from build123d import *

# Parameters (mm, degrees)
F0_W      = 189.7254064679
F0_H      = 125.3468897194
F1_DEPTH  = 3.81
F2_W      = 6.9400146604
F2_H      = 125.3468897194
F3_DEPTH  = 50.8
F4_W      = 7.941737771
F4_H      = 125.3468897194
F5_DEPTH  = 50.8
F6_W      = 181.0236349702
F6_H      = 7.8539922833
F7_DEPTH  = 177.8
F8_W      = 6.9400146604
F8_H      = 66.6004410014
F9_DEPTH  = 50.8
F10_W     = 6.9400146604
F10_H     = 25.5400016904
F11_DEPTH = 76.2
F12_W     = 7.941737771
F12_H     = 58.746448718
F13_DEPTH = 50.8
F14_W     = 6.1799809337
F14_H     = 15.7597959042
F15_DEPTH = 76.2
F16_W     = 189.6112561226
F16_H     = 127.5956835598
F17_DEPTH = 3.302
F18_W     = 1.9466541708
F18_H     = 54.61
F19_DEPTH = 117.602
F20_W     = 11.5141570568
F20_H     = 125.3468897194
F21_DEPTH = 127
F22_W     = 10.0032910705
F22_H     = 125.3468897194
F23_DEPTH = 127
F24_W     = 178.803190589
F24_H     = 6.9889426231
F25_DEPTH = 127


with BuildPart() as f1:
    # F0 (on Top) → F1 (new body)
    with BuildSketch(Plane.XY):
        with Locations((-30.9122316539, 52.4606974795)):
            Rectangle(F0_W, F0_H)
    extrude(amount=F1_DEPTH)

    # F2 (on face) → F3 (join)
    with BuildSketch(Plane.XY.offset(3.81)):
        with Locations((-122.3049275577, 52.4606974795)):
            Rectangle(F2_W, F2_H)
    extrude(amount=F3_DEPTH)

    # F4 (on face) → F5 (join)
    with BuildSketch(Plane.XY.offset(3.81)):
        with Locations((59.9796026945, 52.4606974795)):
            Rectangle(F4_W, F4_H)
    extrude(amount=F5_DEPTH)

    # F6 (on face) → F7 (join)
    with BuildSketch(Plane.XY.offset(3.81)):
        with Locations((-28.3231027424, 111.2071461976)):
            Rectangle(F6_W, F6_H)
    extrude(amount=F7_DEPTH)

    # F8 (on face) → F9 (join)
    with BuildSketch(Plane.XY.offset(54.61)):
        with Locations((-122.3049275577, 81.8339218386)):
            Rectangle(F8_W, F8_H)
    extrude(amount=F9_DEPTH)

    # F10 (on face) → F11 (join)
    with BuildSketch(Plane.XY.offset(105.41)):
        with Locations((-122.3049275577, 102.364141494)):
            Rectangle(F10_W, F10_H)
    extrude(amount=F11_DEPTH)

    # F12 (on face) → F13 (join)
    with BuildSketch(Plane.XY.offset(54.61)):
        with Locations((59.9796026945, 77.9069256969)):
            Rectangle(F12_W, F12_H)
    extrude(amount=F13_DEPTH)

    # F14 (on face) → F15 (join)
    with BuildSketch(Plane.XY.offset(105.41)):
        with Locations((59.0987242758, 99.4002521038)):
            Rectangle(F14_W, F14_H)
    extrude(amount=F15_DEPTH)

    # F16 (on face) → F17 (join)
    with BuildSketch(Plane.XY.offset(54.61)):
        with Locations((-30.9693068266, 53.5850943998)):
            Rectangle(F16_W, F16_H)
    extrude(amount=F17_DEPTH)

    # F18 (on face) → F19 (join)
    with BuildSketch(Plane.XZ.offset(-107.2801500559)):
        with Locations((-30.4397661239, 27.305)):
            Rectangle(F18_W, F18_H)
    extrude(amount=F19_DEPTH)

    # F20 (on face) → F21 (join)
    with BuildSketch(Plane(origin=(0, 0, 0), x_dir=(1, 0, 0), z_dir=(0, 0, -1))):
        with Locations((-120.0178563595, -52.4606974795)):
            Rectangle(F20_W, F20_H)
    extrude(amount=F21_DEPTH)

    # F22 (on face) → F23 (join)
    with BuildSketch(Plane(origin=(0, 0, 0), x_dir=(1, 0, 0), z_dir=(0, 0, -1))):
        with Locations((58.9488260448, -52.4606974795)):
            Rectangle(F22_W, F22_H)
    extrude(amount=F23_DEPTH)

    # F24 (on face) → F25 (join)
    with BuildSketch(Plane(origin=(0, 0, 0), x_dir=(1, 0, 0), z_dir=(0, 0, -1))):
        with Locations((-35.4544147849, -111.6396710277)):
            Rectangle(F24_W, F24_H)
    extrude(amount=F25_DEPTH)


solid = f1.part
Could you check a few things on this model? Use its own coordinates, in mm. A direction names the side the tool comes from. Give positions to 0.01 mm unless a question says otherwise; leave off trailing zeros. Order: outer loops, then holes, each group sorted by start corner. A loop starts at its lowest first (then second) coordinate and runs counter-clockwise, first axis right, second up.
Item 1: I need wall thicknesses on line 1 (X direction, y = 107, z = 20); line 2 (Z direction, x = 24, y = 67); line 3 (X direction, y = 39.5, z = -38.5). Which ranges of each line are inside material? Lowest first, please.
Item 2: If we mould it in two halves opening along Z, with no side actions, what happens to faces 6 (the face through (-31.413, 49, 33)), 7 (the face through (-118.835, 84, 105)), 8 (the face through (-31, 50, 0))? For each: pulls with the +Z half, pulls with the -Z half, needs draft (parallel to the pull), parting line crosses it, or undercut.
Item 3: If we section it at B-B, the plane z = 109: Write out the boundary of the cut face in (x, y).
Item 4: If we section it at C-C, the plane x = 4: Write out the boundary of the cut face in (y, z).
Item 5: If we section it at A-A, the plane y = 15: Write out the boundary of the cut face in (x, z), plus the area to 3 significant figures.
Item 6: For faces 1 (the face through (56.009, 84, 91)), 2 (the face through (-122, 69, 105.41)), 3 (the face through (-76, 49, 3.81)), 4 (the face through (-33, 115.134, 119)), 5 (the face through (-31, 108.145, -63)), which set-ups out of +Z, -Z, +X, -X, +Y, -Y let a thin tool reach every point of the face, with its end or its side?
Item 7: If we section it at D-D, the plane z = -92: Write out the boundary of the cut face in (x, y), plus the area to 3 significant figures.
Item 8: I'm going to push flat-ended pins straight in: pin 1 (1.5 mm diameter, centred on x = -95.5, y = 9.5, fed in from +Z); pin 2 (1.9 mm diameter, centred on x = 63, z = 73, fed in from +Y); pin 3 (7.5 mm diameter, centred on x = -123.5, z = 88, fed in from -Y). Where does each tip first touch, or does it pass through?
Values:
1. line 1: x = -125.77 to -118.83, -31.41 to -29.47, 56.01 to 63.95
1. line 2: z = 0 to 3.81, 54.61 to 57.91
1. line 3: x = -125.77 to -114.26, 53.95 to 63.95
2. face 6: undercut
2. face 7: needs draft
2. face 8: pulls with the -Z half
3. outline: (-125.77, 89.59) - (-118.83, 89.59) - (-118.83, 107.28) - (56.01, 107.28) - (56.01, 91.52) - (62.19, 91.52) - (62.19, 115.13) - (-125.77, 115.13) - close
4. outline: (-10.21, 0) - (108.15, 0) - (108.15, -127) - (115.13, -127) - (115.13, 54.61) - (117.38, 54.61) - (117.38, 57.91) - (115.13, 57.91) - (115.13, 181.61) - (107.28, 181.61) - (107.28, 57.91) - (-10.21, 57.91) - (-10.21, 54.61) - (107.28, 54.61) - (107.28, 3.81) - (-10.21, 3.81) - close
5. outline: (-125.77, -127) - (-114.26, -127) - (-114.26, 0) - (53.95, 0) - (53.95, -127) - (63.95, -127) - (63.95, 54.61) - (63.84, 54.61) - (63.84, 57.91) - (-125.77, 57.91) - close; hole (-118.83, 3.81) - (-31.41, 3.81) - (-31.41, 54.61) - (-118.83, 54.61) - close; hole (-29.47, 3.81) - (56.01, 3.81) - (56.01, 54.61) - (-29.47, 54.61) - close
5. area: 4,940 mm2
6. face 1: +Z, -Y
6. face 2: +Z, +X, -X, -Y
6. face 3: -Y
6. face 4: +Z, +X, -X, +Y
6. face 5: -Z, -Y
7. outline: (-125.77, -10.21) - (-114.26, -10.21) - (-114.26, 108.15) - (53.95, 108.15) - (53.95, -10.21) - (63.95, -10.21) - (63.95, 115.13) - (-125.77, 115.13) - close
7. area: 3,870 mm2
8. pin 1: stops at z = 57.91
8. pin 2: stops at y = 115.13
8. pin 3: stops at y = 48.53
